Build history of the part. All positions in model axes, mm. A direction names the side the tool comes from. Coordinates: 2 decimals unless noted, no trailing zeros. Order: outer loops, then holes, each group sorted by start corner. A loop starts at its lowest first (then second) coordinate and runs counter-clockwise, first axis right, second up. Notation, with made-up numbers: (27.5, 68.5) - (66.5, 68.5) arc R4 cw to (66.5, 73.5) - close; hole circle Ø11 at (81, 87.25). An arc over 180 degrees is marked (long way). Return JSON: item names as keys, results as strings.
from build123d import *

# Parameters (mm, degrees)
SKETCH1_W           = 66
SKETCH1_H           = 15
BOSS_EXTRUDE1_DEPTH = 6
SKETCH2_W           = 35
SKETCH2_H           = 15
BOSS_EXTRUDE2_DEPTH = 29
FILLET1_R           = 17.5
SKETCH3_R           = 7
BOSS_EXTRUDE3_DEPTH = 4
SKETCH4_R           = 5
CUT_EXTRUDE1_DEPTH  = 52.720402164
SKETCH5_R           = 3
CUT_EXTRUDE2_DEPTH  = 46.412002819


with BuildPart() as part:
    # Sketch1 → Boss-Extrude1 (new body)
    with BuildSketch(Plane(origin=(0, 0, 0), x_dir=(1, 0, 0), z_dir=(0, 1, 0))):
        Rectangle(SKETCH1_W, SKETCH1_H)
    extrude(amount=BOSS_EXTRUDE1_DEPTH)

    # Sketch2 → Boss-Extrude2 (add)
    with BuildSketch(Plane(origin=(0, 6, 0), x_dir=(1, 0, 0), z_dir=(0, 1, 0))):
        Rectangle(SKETCH2_W, SKETCH2_H)
    extrude(amount=BOSS_EXTRUDE2_DEPTH)

    # Fillet1
    fillet1_edges = [part.edges().sort_by_distance(p)[0] for p in [
        (17.5, 35, 0),
        (-17.5, 35, 0),
    ]]
    fillet(fillet1_edges, radius=FILLET1_R - 0.0001)  # a hair under: the kernel refuses the full size

    # Sketch3 → Boss-Extrude3 (add)
    with BuildSketch(Plane.XY.offset(7.5)):
        with Locations(Location((0, 17.5, 0), (0, 0, 180))):
            Circle(SKETCH3_R)
    extrude(amount=BOSS_EXTRUDE3_DEPTH)

    # Sketch4 → Cut-Extrude1 (cut, through all)
    with BuildSketch(Plane.XY.offset(11.5)):
        with Locations((0, 17.5)):
            Circle(SKETCH4_R)
    extrude(amount=-CUT_EXTRUDE1_DEPTH, mode=Mode.SUBTRACT)

    # Sketch5 → Cut-Extrude2 (cut, through all)
    with BuildSketch(Plane(origin=(0, 6, 0), x_dir=(1, 0, 0), z_dir=(0, 1, 0))):
        with Locations(Location((-27, 0, 0), (0, 0, 270))):
            Circle(SKETCH5_R)
    cut_extrude2 = extrude(amount=-CUT_EXTRUDE2_DEPTH, mode=Mode.SUBTRACT)

    # Mirror1: Cut-Extrude2 across plane
    add(cut_extrude2.mirror(Plane(origin=(0, 0, 0), x_dir=(0, 0, 1), z_dir=(1, 0, 0))), mode=Mode.SUBTRACT)


solid = part.part
1. Mould opens along Z. For faces 4 (the cylindrical face through (-26.1, 3.04, 2.86)), 5 (the flat face through (0, 9, 7.5)), 6 (the cylindrical face through (1.517, 24.334, 9.472)), 7 (the cylindrical face through (26.1, 3.04, 2.86)) say: pulls with the +Z half, pulls with the -Z half, needs draft (parallel to the pull), parting line crosses it, or undercut.
Check values:
{"face 4": "undercut", "face 5": "pulls with the +Z half", "face 6": "needs draft", "face 7": "undercut"}
2. Cut at D-D on y = 19. Give the cut face in (x, z), plus the area to 3 significant figures.
Check values:
{"outline": "(-17.44, -7.5) - (-4.77, -7.5) - (-4.77, 11.5) - (-6.84, 11.5) - (-6.84, 7.5) - (-17.44, 7.5) - close; (4.77, -7.5) - (17.44, -7.5) - (17.44, 7.5) - (6.84, 7.5) - (6.84, 11.5) - (4.77, 11.5) - close", "area": "397 mm²"}
3. Tool access for faces 1 (the flat face through (-23.6, 6, -0.1)), 2 (the flat face through (-33, 3, 0)), 3 (the flat face through (17.5, 12, 0)): list every direction of +Z, -Z, +X, -X, +Y, -Y with a clear straight run to the whole face (end or side of a thin tool).
Check values:
{"face 1": "+Z, -Z, -X, +Y", "face 2": "+Z, -Z, -X, +Y, -Y", "face 3": "+Z, -Z, +X, +Y"}
4. Drop flat-ended pins along their axis: pin 1 (1.5 mm diameter, centred on y = 17, z = 2, fed in from +X); pin 2 (4.5 mm diameter, centred on x = 24.5, z = -3.5, fed in from +Y). Give the stop position or say it passes through.
Check values:
{"pin 1": "x = 17.5", "pin 2": "y = 6"}
5. Cut at B-B on x = -27. Give the cut face in (y, z).
Check values:
{"outline": "(0, -7.5) - (6, -7.5) - (6, -3) - (0, -3) - close; (0, 3) - (6, 3) - (6, 7.5) - (0, 7.5) - close"}
6. Probe L1, parallel to X at y = 4.5, z = 0.25; L2, parallel to Y at x = 0, z = 2.5; L3, parallel to X at y = 13.5, z = -5.5. List the from-to ranges inside material, lowest first.
Check values:
{"L1": "-33 to -29.99, -24.01 to 24.01, 29.99 to 33", "L2": "0 to 12.5, 22.5 to 35", "L3": "-17.5 to -3, 3 to 17.5"}
7. Cut at A-A on z = 0. State how many separate pieces and enclosed holes the cut face has, plus the area to 3 significant figures.
Check values:
{"separate pieces": "3", "enclosed holes": "1", "area": "1,130 mm²"}
